Verification items for the finished model (mm, model axes). Face numbers are marked on the shaded views. A direction names the side the tool comes from. Give positions to 0.01 mm unless a question says otherwise; leave off trailing zeros. Loops run counter-clockwise (first coordinate to the right, second up) from the corner with the lowest first, then second, coordinate; pieces in that order, holes last. Notation, with made-up numbers: M -36.5,50.25 L -31.5,50.25 A20 ccw -31.5,85.25 Z; hole C 82,73 d11. An arc over 180 degrees is marked long. Put each result on its own line as item: value. Start each with the question number.
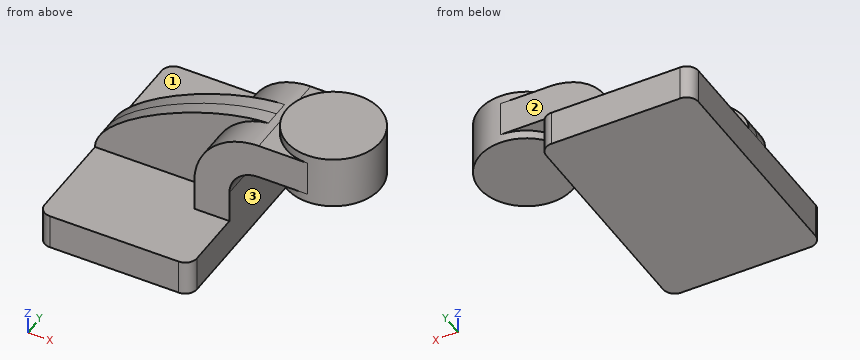
from build123d import *

# Parameters (mm, degrees)
F1_DEPTH = 63.5
F0_W     = 25.4
F0_H     = 19.05
F2_DEPTH = 25.4
F3_DEPTH = 7.9375
F5_R     = 6.35


with BuildPart() as f1:
    # F0 (on Front) → F1 (new body, symmetric)
    with BuildSketch(Plane.XZ):
        Polygon((-41.275, 9.525), (-41.275, -9.525), (41.275, -9.525), (41.275, 9.525), (22.225, 9.525), align=None)
    extrude(amount=F1_DEPTH, both=True)

    # F0 (on Front) → F2 (join, symmetric)
    with BuildSketch(Plane.XZ):
        with BuildLine():
            Line((22.225, 9.525), (41.275, 9.525))
            Line((41.275, 9.525), (41.275, 27.00782))
            ThreePointArc((41.275, 27.00782), (45.9246798487, 38.2331401513), (57.15, 42.88282))
            Line((57.15, 42.88282), (58.1977560132, 42.88282))
            Line((58.1977560132, 42.88282), (58.1977560132, 61.93282))
            Line((58.1977560132, 61.93282), (57.15, 61.93282))
            ThreePointArc((57.15, 61.93282), (54.9328944769, 61.862375916), (52.724732803, 61.6513278368))
            ThreePointArc((52.724732803, 61.6513278368), (30.9363768066, 50.0859824934), (22.225, 27.00782))
            Line((22.225, 27.00782), (22.225, 9.525))
        make_face()
        with Locations((70.8977560132, 52.40782)):
            Rectangle(F0_W, F0_H)
    extrude(amount=F2_DEPTH, both=True)

    # F0 (on Front) → F3 (join, symmetric)
    with BuildSketch(Plane.XZ):
        with BuildLine():
            add(Edge.make_bspline(
                [(-41.275, 9.525), (-41.5120311081, 29.9139209092), (17.1590354294, 60.4301430285), (52.724732803, 61.6513278368)],
                knots=[0, 0, 0, 0, 107.4853656122, 107.4853656122, 107.4853656122, 107.4853656122], degree=3))
            Line((-41.275, 9.525), (22.225, 9.525))
            Line((22.225, 9.525), (22.225, 27.00782))
            ThreePointArc((22.225, 27.00782), (30.9363768066, 50.0859824934), (52.724732803, 61.6513278368))
        make_face()
    extrude(amount=F3_DEPTH, both=True)

    # F0 (on Front) → F4 (revolve)
    with BuildSketch(Plane.XZ):
        Polygon((83.5977560132, 66.675), (83.5977560132, 61.93282), (83.5977560132, 42.88282), (83.5977560132, 38.1), (108.9977560132, 38.1), (108.9977560132, 66.675), align=None)
    revolve(axis=Axis((83.5977560132, 0, 52.3875), (0, 0, 1)))

    # F5
    f5_edges = [f1.edges().sort_by_distance(p)[0] for p in [
        (41.275, -63.5, 0),
        (-41.275, -63.5, 0),
        (41.275, 63.5, 0),
        (-41.275, 63.5, 0),
    ]]
    fillet(f5_edges, radius=F5_R)


solid = f1.part
Q1. Scan lines: L1, parallel to Y at x = -19, z = 24; L2, parallel to Z at x = 8.5, y = 46.5 (3 decimals); L3, parallel to Y at x = 46, z = 47. Record each from-to range of solid material in increasing order.
Q2. Cross-section at C-C, the plane x = 86. Record the boundary of the cut face in (y, z) (3 decimals), then the cut area to 3 significant figures.
Q3. Go/stop test with flat-tipped pins: pin 1 (4 mm diameter, centred on x = 89, z = 44, fed in from +Y); pin 2 (4 mm diameter, centred on x = -3, y = -3.5, fed in from +Z); pin 3 (1 mm diameter, centred on x = -6.5, z = 15, fed in from +Y); pin 4 (6 mm diameter, centred on x = 61.5, y = -30, fed in from +Z). Record where each tip stops, or that it passes through.
Q4. Cross-section at D-D, the plane y = -44. Record the boundary of the cut face in (x, z) (3 decimals).
Q5. Cross-section at B-B, the plane y = -14.5. Record the boundary of the cut face in (x, z) (3 decimals).
Q6. Set-up check for the marked faces 1, 2 and 3: record each of +Z, -Z, +X, -X, +Y, -Y from which the full face is reachable in a straight line by a thin tool's end or side.
Q7. Cross-section at A-A, the plane z = 3. Record the boundary of the cut face in (x, y) (3 decimals).
Ans:
1. L1: y = -7.94 to 7.94
1. L2: z = -9.525 to 9.525
1. L3: y = -25.4 to 25.4
2. outline: M -25.286,38.1 L 25.286,38.1 L 25.286,66.675 L -25.286,66.675 Z
2. area: 1,450 mm^2
3. pin 1: stops at y = 25.17
3. pin 2: stops at z = 46.22
3. pin 3: stops at y = 7.94
3. pin 4: passes through
4. outline: M -41.275,-9.525 L 41.275,-9.525 L 41.275,9.525 L -41.275,9.525 Z
5. outline: M -41.275,-9.525 L 41.275,-9.525 L 41.275,27.008 A15.875 cw 57.15,42.883 L 62.743,42.883 L 62.743,38.1 L 104.452,38.1 L 104.452,66.675 L 62.743,66.675 L 62.743,61.933 L 57.15,61.933 A34.925 ccw 22.225,27.008 L 22.225,9.525 L -41.275,9.525 Z
6. face 1: +Z, -X, +Y
6. face 2: +Z, +X, -X, +Y
6. face 3: -Z, +X, +Y, -Y
7. outline: M -41.275,-57.15 A6.35 ccw -34.925,-63.5 L 34.925,-63.5 A6.35 ccw 41.275,-57.15 L 41.275,57.15 A6.35 ccw 34.925,63.5 L -34.925,63.5 A6.35 ccw -41.275,57.15 Z
